Autodesk Inventor part; units mm, degrees
ref_plane "Start Plane" through (0, 0, 0) normal (0, 0, 1) x (1, 0, 0)
ref_plane "End Plane" through (0, 0, 50) normal (0, 0, 1) x (1, 0, 0)
ref_plane "Work Plane4" through (0, 12.7, 50) normal (0.7071, 0, 0.7071) x (0.7071, 0, -0.7071)
ref_plane "Start Plane" through (0, 0, 0) normal (0, 0, 1) x (1, 0, 0)
ref_plane "End Plane" through (0, 0, 50) normal (0, 0, 1) x (1, 0, 0)
sketch "Sketch" plane through (0, 0, 0) normal (0, 0, 1) x (1, 0, 0)
  line L0 (25.4, 0) -> (0, 0)
  line L1 (0, 0) -> (0, 25.4)
  line L2 (0, 25.4) -> (1.651, 25.4)
  line L3 (3.175, 23.876) -> (3.175, 6.477)
  line L4 (6.477, 3.175) -> (23.876, 3.175)
  line L5 (25.4, 1.651) -> (25.4, 0)
  line L6 (0, -11.0414) -> (0, 31.5385) construction
  line L7 (-11.0414, 0) -> (31.5385, 0) construction
  arc A0 (3.175, 6.477) -> (6.477, 3.175) centre (6.477, 6.477) ccw
  arc A1 (3.175, 23.876) -> (1.651, 25.4) centre (1.651, 23.876) ccw
  arc A2 (25.4, 1.651) -> (23.876, 3.175) centre (23.876, 1.651) ccw
  line L8 (0, 40.0545) -> (0, -19.5574) construction
  line L9 (-19.5574, 0) -> (40.0545, 0) construction
  point P0 (3.175, 25.4)
  point P1 (3.175, 3.175)
  point P2 (25.4, 3.175)
  dimension "d0" = 25.4
  dimension "d1" = 25.4
  dimension "d2" = 3.175
  dimension "d3" = 3.175
  dimension "d10" = 0
  dimension "d11" = 0
  dimension "d14" = 3.302
  dimension "d15" = 1.524
extrude "Body" add sketch "Sketch" along normal up to surface (50 mm away) from surface at 0
sketch "Sketch3" plane through (0, 0, 0) normal (0, 0, 1) x (1, 0, 0)
  line L0 (0, 0) -> (10, 0)
ref_plane "Work Plane3" through (0, 0, 0) normal (0, -1, 0) x (1, 0, 0)
ref_plane "Work Plane4" through (0, 12.7, 50) normal (0.7071, 0, 0.7071) x (0.7071, 0, -0.7071)
split "Split1" plane through (0, 12.7, 50) removes the side toward (0.7071, 0, 0.7071)
ref_plane "Work Plane5" through (12.7, 0, 0) normal (0, 0.3827, -0.9239) x (1, 0, 0)
split "Split2" plane through (12.7, 0, 0) removes the side toward (0, 0.3827, -0.9239)
sketch "Sketch4" plane through (0, 0, 0) normal (0, -1, 0) x (1, 0, 0)
  line L0 (-2, 0) -> (12, 0)
  line L1 (-2, 50) -> (12, 50)
  dimension "d17" = 50
equation "\"d0\" = G_H"
equation "\"d1\" = G_H"
equation "\"d2\" = G_T"
equation "\"d3\" = G_T"
equation "\"d14\" = G_IR"
equation "\"d15\" = G_ER"
equation "\"d4\" = G_L"
equation "\"G_H\" = 25.4"
equation "\"G_T\" = 3.175"
equation "\"G_ER\" = 1.524"
equation "\"G_IR\" = 3.302"
equation "\"G_L\" = d17"
equation "\"ex\" = 0"
equation "\"G_OFFSET_START\" = 0"
equation "\"G_OFFSET_END\" = 0"
equation "\"d13\" = G_OFFSET_END + B_L"
equation "\"B_L\" = 50"
properties part number "AISC - L 1 x 1 x 1/8 - 1.969" material "Steel, Mild"
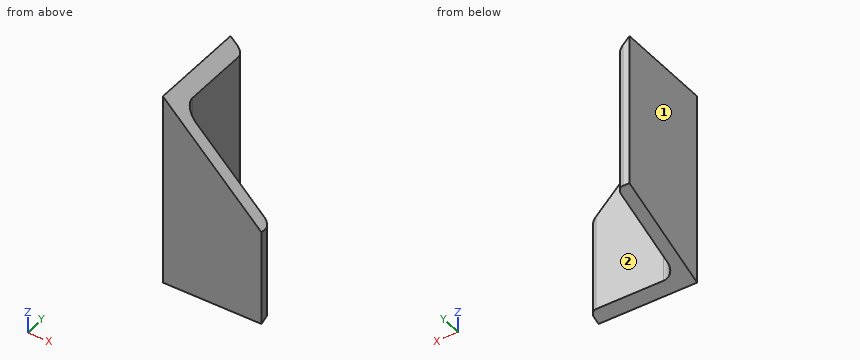
Geometry check sheet. Reference: the model listing, model coordinates, mm. Face numbers are marked on the shaded views. A direction names the side the tool comes from. Coordinates: 2 decimals unless noted, no trailing zeros. Loops run counter-clockwise (first coordinate to the right, second up) from the corner with the lowest first, then second, coordinate; pieces in that order, holes last. Notation, with made-up numbers: (-37.75, 23.25) -> (-3.75, 23.25) arc R25 ccw to (-3.75, 51.25) -> close; hole circle Ø11 at (-16, -22). An arc over 180 degrees is marked (long way). Put each result on its own line as item: value.
1) Cross-section at C-C on y = 14.75. Record the boundary of the cut face in (x, z) (3 decimals), plus the area to 3 significant figures.
Result set:
outline: (0, 6.11) -> (3.175, 6.11) -> (3.175, 46.825) -> (0, 50) -> close
area: 134 mm^2
2) Thickness scan on line 1 (Y direction, x = 14.5, z = 31) (3 decimals); line 2 (Y direction, x = 4.5, z = 5). Record the ranges inside material, lowest first.
Result set:
line 1: y = 0 to 3.175
line 2: y = 0 to 3.83
3) Cross-section at B-B on x = 15. Record the boundary of the cut face in (y, z) (3 decimals).
Result set:
outline: (0, 0) -> (3.175, 1.315) -> (3.175, 35) -> (0, 35) -> close
4) Gauge pin test, flat ends, axial feed: pin 1 Ø10 at (x, y) = (17.5, 11.5) entering from +Z; pin 2 Ø5 at (y, z) = (20, 16) entering from +X (3 decimals); pin 3 Ø2 at (y, z) = (19, 41) entering from -X; pin 4 Ø8.5 at (x, z) = (13, 21.5) entering from +Y (3 decimals). Record the tip position at first contact, or that the pin passes through.
Result set:
pin 1: passes through
pin 2: stops at x = 3.175
pin 3: stops at x = 0
pin 4: stops at y = 3.175
5) Cross-section at D-D on z = 19.5. Record the boundary of the cut face in (x, y) (3 decimals).
Result set:
outline: (0, 0) -> (25.4, 0) -> (25.4, 1.651) arc R1.524 ccw to (23.876, 3.175) -> (6.477, 3.175) arc R3.302 cw to (3.175, 6.477) -> (3.175, 23.876) arc R1.524 ccw to (1.651, 25.4) -> (0, 25.4) -> close
6) Tool access check on the marked faces 1 and 2. Record the directions out of +Z, -Z, +X, -X, +Y, -Y that give a thin tool (end or side, any length) a straight path to the whole face; none if there is none.
Result set:
face 1: +Z, -Z, -X, +Y, -Y
face 2: +Z, -Z, +X, +Y
7) Cross-section at A-A on z = 35. Record the boundary of the cut face in (x, y) (3 decimals).
Result set:
outline: (0, 0) -> (15, 0) -> (15, 3.175) -> (6.477, 3.175) arc R3.302 cw to (3.175, 6.477) -> (3.175, 23.876) arc R1.524 ccw to (1.651, 25.4) -> (0, 25.4) -> close
